Part print with two shaded views. Sizes in mm from the minimum x, y, z corner. Coordinates: 2 decimals unless noted, no trailing zeros. Order: outer loops, then holes, each group sorted by start corner. A loop starts at its lowest first (then second) coordinate and runs counter-clockwise, first axis right, second up. Notation, with made-up numbers: (77.25, 77) - (110.25, 77) arc R26 cw to (110.25, 103) - close; hole circle Ø5 at (68.5, 38). An arc over 180 degrees is marked (long way). One line per item, written item: value.
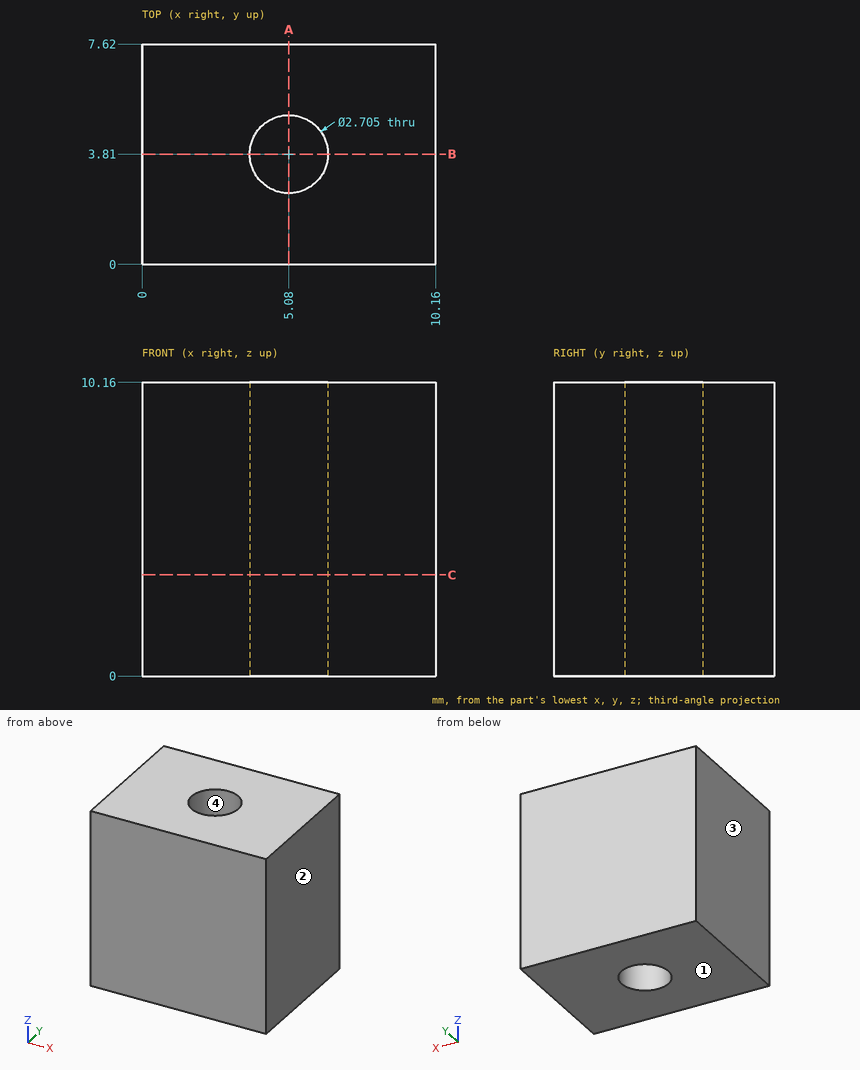
1. Two-plate mould, pull along X, no slides. Class the marked faces 1, 2, 3 and 4: pulls with the +X half, pulls with the -X half, needs draft (parallel to the pull), parting line crosses it, or undercut.
Values found:
face 1: needs draft
face 2: pulls with the +X half
face 3: pulls with the -X half
face 4: undercut
2. Band-saw the part on B-B, the plane y = 3.81. Give the cut face in (x, z).
Values found:
outline: (0, 0) - (3.73, 0) - (3.73, 10.16) - (0, 10.16) - close; (6.43, 0) - (10.16, 0) - (10.16, 10.16) - (6.43, 10.16) - close
3. Band-saw the part on A-A, the plane x = 5.08. Give the cut face in (y, z).
Values found:
outline: (0, 0) - (2.46, 0) - (2.46, 10.16) - (0, 10.16) - close; (5.16, 0) - (7.62, 0) - (7.62, 10.16) - (5.16, 10.16) - close
4. Probe line 1 along Y through (x, z) = (5.08, 6); line 2 along X through (y, z) = (3.25, 6.5); line 3 along Y through (x, z) = (6.25, 8.25). List the from-to ranges inside material, lowest first.
Values found:
line 1: y = 0 to 2.46, 5.16 to 7.62
line 2: x = 0 to 3.85, 6.31 to 10.16
line 3: y = 0 to 3.13, 4.49 to 7.62
5. Band-saw the part on C-C, the plane z = 3.5. Give the cut face in (x, y) (1 decimal), and give its area (3 significant figures).
Values found:
outline: (0, 0) - (10.2, 0) - (10.2, 7.6) - (0, 7.6) - close; hole circle Ø2.7 at (5.1, 3.8)
area: 71.7 mm2
